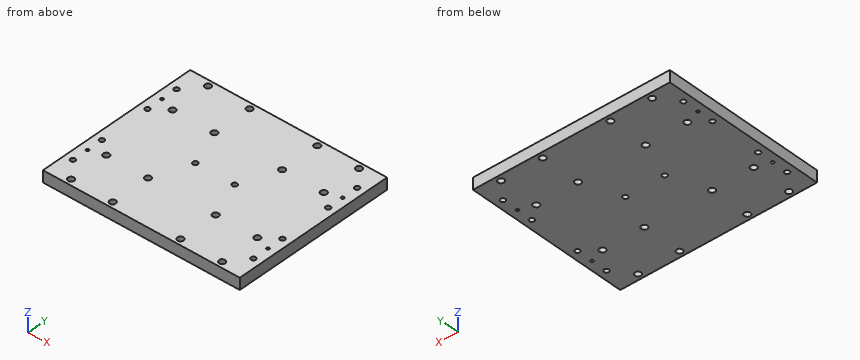
from build123d import *

# Parameters (mm, degrees)
SKETCH1_W                      = 170
SKETCH1_H                      = 142
BOSS_EXTRUDE1_DEPTH            = 5
M5_CLEARANCE_HOLE1_D           = 5.3
MIRROR3_COPY_1_D               = 5.3
M4_CLEARANCE_HOLE1_D           = 4.3
M5X0_8_TAPPED_HOLE1_AT_2_COUNT = 2
M5X0_8_TAPPED_HOLE1_AT_2_PITCH = 28
SKETCH6_R                      = 1.25
CUT_EXTRUDE5_DEPTH             = 11
MIRROR4_COPY_2_SKETCH_R        = 1.25
MIRROR4_COPY_2_DEPTH           = 11


with BuildPart() as part:
    # Sketch1 → Boss-Extrude1 (new body, symmetric)
    with BuildSketch(Plane.XY):
        Rectangle(SKETCH1_W, SKETCH1_H)
    extrude(amount=BOSS_EXTRUDE1_DEPTH, both=True)

    # M5 Clearance Hole1 (through all)
    with Locations(Plane.XY.offset(5)):
        with Locations((-65.25, 66), (-29.25, 66), (-29.25, 32), (-65.25, 32)):
            m5_clearance_hole1 = Hole(M5_CLEARANCE_HOLE1_D / 2)

    # Mirror2: M5 Clearance Hole1 across plane
    add(m5_clearance_hole1.mirror(Plane.ZX), mode=Mode.SUBTRACT)

    # Mirror3: M5 Clearance Hole1 across plane
    add(m5_clearance_hole1.mirror(Plane(origin=(0, 0, 0), x_dir=(0, 0, 1), z_dir=(1, 0, 0))), mode=Mode.SUBTRACT)

    # Mirror3 copy 1 (through all)
    with Locations(Plane(origin=(0, 0, 5), x_dir=(-1, 0, 0), z_dir=(0, 0, 1))):
        with Locations((-65.25, 66), (-29.25, 66), (-29.25, 32), (-65.25, 32)):
            Hole(MIRROR3_COPY_1_D / 2)

    # M4 Clearance Hole1 (through all)
    with Locations(Plane.XY.offset(5)):
        with Locations((-17, 0), (17, 0)):
            Hole(M4_CLEARANCE_HOLE1_D / 2)

    # Sketch11 → M5x0.8 Tapped Hole1 (revolve, cut)
    with BuildSketch(Plane(origin=(-78, 50, 5), x_dir=(0, -1, 0), z_dir=(1, 0, 0))):
        Polygon((0, 0), (0, 15.2618073), (2.1, 14), (2.1, 0), align=None)
    m5x0_8_tapped_hole1 = revolve(axis=Axis((-78, 50, 11.35), (0, 0, -1)), mode=Mode.SUBTRACT)

    # M5x0.8 Tapped Hole1 at 2: M5x0.8 Tapped Hole1 ×2
    with Locations(*[(0, -i * M5X0_8_TAPPED_HOLE1_AT_2_PITCH, 0) for i in range(1, M5X0_8_TAPPED_HOLE1_AT_2_COUNT)]):
        add(m5x0_8_tapped_hole1, mode=Mode.SUBTRACT)

    # Sketch6 → Cut-Extrude5 (cut, through all)
    with BuildSketch(Plane.XY.offset(5)):
        with Locations((-78, 36)):
            Circle(SKETCH6_R)
    cut_extrude5 = extrude(amount=-CUT_EXTRUDE5_DEPTH, mode=Mode.SUBTRACT)

    # Mirror1: M5x0.8 Tapped Hole1, Cut-Extrude5 across plane
    add(m5x0_8_tapped_hole1.mirror(Plane(origin=(0, 0, 0), x_dir=(0, 0, 1), z_dir=(1, 0, 0))), mode=Mode.SUBTRACT)
    add(cut_extrude5.mirror(Plane(origin=(0, 0, 0), x_dir=(0, 0, 1), z_dir=(1, 0, 0))), mode=Mode.SUBTRACT)

    # Mirror1 copy 1 sketch → Mirror1 copy 1 (revolve, cut)
    with BuildSketch(Plane(origin=(78, 22, 5), x_dir=(0, -1, 0), z_dir=(-1, 0, 0))):
        Polygon((0, 0), (0, -15.2618073), (2.1, -14), (2.1, 0), align=None)
    revolve(axis=Axis((78, 22, 11.35), (0, 0, 1)), mode=Mode.SUBTRACT)

    # Mirror4: M5x0.8 Tapped Hole1, Cut-Extrude5 across plane
    add(m5x0_8_tapped_hole1.mirror(Plane.ZX), mode=Mode.SUBTRACT)
    add(cut_extrude5.mirror(Plane.ZX), mode=Mode.SUBTRACT)

    # Mirror4 copy 1 sketch → Mirror4 copy 1 (revolve, cut)
    with BuildSketch(Plane(origin=(78, -50, 5), x_dir=(0, 1, 0), z_dir=(-1, 0, 0))):
        Polygon((0, 0), (0, 15.2618073), (2.1, 14), (2.1, 0), align=None)
    revolve(axis=Axis((78, -50, 11.35), (0, 0, -1)), mode=Mode.SUBTRACT)

    # Mirror4 copy 2 sketch → Mirror4 copy 2 (cut, through all)
    with BuildSketch(Plane(origin=(0, 0, 5), x_dir=(-1, 0, 0), z_dir=(0, 0, 1))):
        with Locations((-78, 36)):
            Circle(MIRROR4_COPY_2_SKETCH_R)
    extrude(amount=-MIRROR4_COPY_2_DEPTH, mode=Mode.SUBTRACT)

    # Mirror4 copy 3 sketch → Mirror4 copy 3 (revolve, cut)
    with BuildSketch(Plane(origin=(78, -22, 5), x_dir=(0, 1, 0), z_dir=(-1, 0, 0))):
        Polygon((0, 0), (0, 15.2618073), (2.1, 14), (2.1, 0), align=None)
    revolve(axis=Axis((78, -22, 11.35), (0, 0, -1)), mode=Mode.SUBTRACT)

    # Mirror4 copy 4 sketch → Mirror4 copy 4 (revolve, cut)
    with BuildSketch(Plane(origin=(-78, -22, 5), x_dir=(0, 1, 0), z_dir=(1, 0, 0))):
        Polygon((0, 0), (0, -15.2618073), (2.1, -14), (2.1, 0), align=None)
    revolve(axis=Axis((-78, -22, 11.35), (0, 0, 1)), mode=Mode.SUBTRACT)


solid = part.part
CAD build for the part. Positions are in the model's coordinates, mm. Give positions to 0.01 mm unless a question says otherwise; leave off trailing zeros. Write each loop counter-clockwise with the first axis right and the second up, starting at its lowest first coordinate (ties: lowest second). Pieces come first, ordered by that corner, then holes. Notation, with made-up numbers: M -6,87.5 L 10,87.5 A31 cw 10,119.5 Z; hole C 71,-21 d6. An arc over 180 degrees is marked long. Put each result on its own line as item: value. Start each with the question number.
(1) Band-saw the part on A-A, the plane y = 0. Write the cut outline in (x, z), and give its area (3 significant figures).
(2) Probe L1, parallel to Y at x = 65.25, z = -1.75; L2, parallel to X at y = -50, z = 0.75; L3, parallel to X at y = -36, z = 0. List the from-to ranges inside material, lowest first.
(3) Band-saw the part on C-C, the plane z = 1.5. Give the number of separate pieces and of enclosed holes in the cut face, and give its area (3 significant figures).
(4) Band-saw the part on D-D, the plane y = -32. Write the cut outline in (x, z), and give its area (3 significant figures).
(5) Flat gauge pin, fed straight in: pin 1 Ø5 at (x, y) = (29.25, 66) entering from -Z. Where does the tip first touch, or does it go through?
(6) Band-saw the part on B-B, the plane x = 29.25. Write the cut outline in (y, z), and give its area (3 significant figures).
Response values:
1. outline: M -85,-5 L -19.15,-5 L -19.15,5 L -85,5 Z; M -14.85,-5 L 14.85,-5 L 14.85,5 L -14.85,5 Z; M 19.15,-5 L 85,-5 L 85,5 L 19.15,5 Z
1. area: 1,610 mm2
2. L1: y = -71 to -68.65, -63.35 to -34.65, -29.35 to 29.35, 34.65 to 63.35, 68.65 to 71
2. L2: x = -85 to -80.1, -75.9 to 75.9, 80.1 to 85
2. L3: x = -85 to -79.25, -76.75 to 76.75, 79.25 to 85
3. separate pieces: 1
3. enclosed holes: 30
3. area: 23,600 mm2
4. outline: M -85,-5 L -67.9,-5 L -67.9,5 L -85,5 Z; M -62.6,-5 L -31.9,-5 L -31.9,5 L -62.6,5 Z; M -26.6,-5 L 26.6,-5 L 26.6,5 L -26.6,5 Z; M 31.9,-5 L 62.6,-5 L 62.6,5 L 31.9,5 Z; M 67.9,-5 L 85,-5 L 85,5 L 67.9,5 Z
4. area: 1,490 mm2
5. pin 1: passes through
6. outline: M -71,-5 L -68.65,-5 L -68.65,5 L -71,5 Z; M -63.35,-5 L -34.65,-5 L -34.65,5 L -63.35,5 Z; M -29.35,-5 L 29.35,-5 L 29.35,5 L -29.35,5 Z; M 34.65,-5 L 63.35,-5 L 63.35,5 L 34.65,5 Z; M 68.65,-5 L 71,-5 L 71,5 L 68.65,5 Z
6. area: 1,210 mm2
